from build123d import *

# Parameters (mm, degrees)
F0_W     = 1016
F0_H     = 381
F0_R     = 6.35
F1_DEPTH = 12.7


with BuildPart() as f1:
    # F0 (on Top) → F1 (new body)
    with BuildSketch(Plane.XY):
        with Locations((124.979544, -16.168576)):
            Rectangle(F0_W, F0_H)
        Polygon((-344.920456, -155.868576), (-344.920456, -16.168576), (-344.920456, 123.531424), (-243.320456, 123.531424), (-243.320456, -155.868576), align=None, mode=Mode.SUBTRACT)
        with Locations((-205.220456, -16.168576)):
            Circle(F0_R, mode=Mode.SUBTRACT)
        with Locations((124.979544, -16.168576)):
            Circle(F0_R, mode=Mode.SUBTRACT)
        with Locations((455.179544, -16.168576)):
            Circle(F0_R, mode=Mode.SUBTRACT)
        Polygon((493.279544, -155.868576), (493.279544, 123.531424), (594.879544, 123.531424), (594.879544, -16.168576), (594.879544, -155.868576), align=None, mode=Mode.SUBTRACT)
    extrude(amount=F1_DEPTH)


solid = f1.part
Here's how the part is built. I have some questions about the finished solid (model axes, mm). Round coordinates to 2 decimals unless told otherwise and drop trailing zeros. Loops run counter-clockwise (first coordinate to the right, second up) from the corner with the lowest first, then second, coordinate; pieces in that order, holes last. Notation, with made-up numbers: M 66,26 L 98,26 A21 ccw 98,64 Z; hole C 43,47 d8. An arc over 180 degrees is marked long. Write each question's results on one line, items separated by ' | '. Start each with the question number.
(1) I want a section at B-B (x = -263.5). Please give me the cut outline in (y, z), then the cut area to 3 significant figures.
(2) I want a section at C-C (z = 7.5). Please give me the cut outline in (x, y).
(3) I want a section at A-A (y = 26). Please give me the cut outline in (x, z).
(4) If I drill on probe 1 along X at (y, z) = (-66, 9); probe 2 along Y at (x, z) = (579, 1); probe 3 along Y at (x, z) = (455.5, 12.25), over which ranges is the centre line in solid material (lowest first)? Write a range as from..to.
Solved:
1) outline: M -206.67,0 L -155.87,0 L -155.87,12.7 L -206.67,12.7 Z; M 123.53,0 L 174.33,0 L 174.33,12.7 L 123.53,12.7 Z | area: 1,290 mm²
2) outline: M -383.02,-206.67 L 632.98,-206.67 L 632.98,174.33 L -383.02,174.33 Z; hole M -344.92,-155.87 L -243.32,-155.87 L -243.32,123.53 L -344.92,123.53 Z; hole C -205.22,-16.17 d12.7; hole C 124.98,-16.17 d12.7; hole C 455.18,-16.17 d12.7; hole M 493.28,-155.87 L 594.88,-155.87 L 594.88,123.53 L 493.28,123.53 Z
3) outline: M -383.02,0 L -344.92,0 L -344.92,12.7 L -383.02,12.7 Z; M -243.32,0 L 493.28,0 L 493.28,12.7 L -243.32,12.7 Z; M 594.88,0 L 632.98,0 L 632.98,12.7 L 594.88,12.7 Z
4) probe 1: x = -383.02..-344.92, -243.32..493.28, 594.88..632.98 | probe 2: y = -206.67..-155.87, 123.53..174.33 | probe 3: y = -206.67..-22.51, -9.83..174.33
